The listing builds one solid part. Answer for the finished solid, in the listing's coordinates (mm). Give positions to 0.01 mm unless a question says otherwise; leave off trailing zeros. Loops run counter-clockwise (first coordinate to the right, second up) from the corner with the lowest first, then second, coordinate; pieces in that order, holes last. Notation, with made-up numbers: (67, 53.25) - (125, 53.25) arc R30 ccw to (125, 92.25) - close; hole circle Ø2 at (46.5, 77). An arc over 180 degrees is marked (long way). Answer in a Markdown table with one row per item. Add a question column.
```python
from build123d import *

# Parameters (mm, degrees)
SKETCH1_W           = 200
SKETCH1_H           = 180
BOSS_EXTRUDE1_DEPTH = 2
SKETCH2_W           = 55
SKETCH2_H           = 50
CUT_EXTRUDE1_DEPTH  = 4
SKETCH3_W           = 30
SKETCH3_H           = 70
CUT_EXTRUDE2_DEPTH  = 16
SKETCH4_R           = 1.5
CUT_EXTRUDE3_DEPTH  = 10
SKETCH5_R           = 1.75
CUT_EXTRUDE4_DEPTH  = 10
SKETCH6_R           = 1.5
CUT_EXTRUDE5_DEPTH  = 2
SKETCH7_R           = 1.15
CUT_EXTRUDE6_DEPTH  = 2
SKETCH8_R           = 1.5
CUT_EXTRUDE7_DEPTH  = 2


with BuildPart() as part:
    # Sketch1 → Boss-Extrude1 (new body)
    with BuildSketch(Plane(origin=(0, 0, 0), x_dir=(1, 0, 0), z_dir=(0, 1, 0))):
        Rectangle(SKETCH1_W, SKETCH1_H)
    extrude(amount=BOSS_EXTRUDE1_DEPTH)

    # Sketch2 → Cut-Extrude1 (cut)
    with BuildSketch(Plane(origin=(0, 2, 0), x_dir=(1, 0, 0), z_dir=(0, 1, 0))):
        with Locations((0.5, -65)):
            Rectangle(SKETCH2_W, SKETCH2_H)
    extrude(amount=-CUT_EXTRUDE1_DEPTH, mode=Mode.SUBTRACT)

    # Sketch3 → Cut-Extrude2 (cut)
    with BuildSketch(Plane(origin=(0, 2, 0), x_dir=(1, 0, 0), z_dir=(0, 1, 0))):
        with Locations((85, 55)):
            Rectangle(SKETCH3_W, SKETCH3_H)
        with Locations((-85, 55)):
            Rectangle(SKETCH3_W, SKETCH3_H)
    extrude(amount=-CUT_EXTRUDE2_DEPTH, mode=Mode.SUBTRACT)

    # Sketch4 → Cut-Extrude3 (cut)
    with BuildSketch(Plane(origin=(0, 2, 0), x_dir=(1, 0, 0), z_dir=(0, 1, 0))):
        with Locations((90, -80)):
            Circle(SKETCH4_R)
        with Locations((-90, -80)):
            Circle(SKETCH4_R)
        with Locations((60, 80)):
            Circle(SKETCH4_R)
        with Locations((-60, 80)):
            Circle(SKETCH4_R)
    extrude(amount=-CUT_EXTRUDE3_DEPTH, mode=Mode.SUBTRACT)

    # Sketch5 → Cut-Extrude4 (cut)
    with BuildSketch(Plane(origin=(0, 2, 0), x_dir=(1, 0, 0), z_dir=(0, 1, 0))):
        with Locations((60, 20)):
            Circle(SKETCH5_R)
        with Locations((22.6, 20)):
            Circle(SKETCH5_R)
        with Locations((22.6, -16.7)):
            Circle(SKETCH5_R)
        with Locations((60, -16.7)):
            Circle(SKETCH5_R)
    extrude(amount=-CUT_EXTRUDE4_DEPTH, mode=Mode.SUBTRACT)

    # Sketch6 → Cut-Extrude5 (cut)
    with BuildSketch(Plane(origin=(0, 2, 0), x_dir=(1, 0, 0), z_dir=(0, 1, 0))):
        with Locations((-95, -60.635083269)):
            Circle(SKETCH6_R)
        with Locations((-95, -18.235083269)):
            Circle(SKETCH6_R)
        with Locations((95, -60.635083269)):
            Circle(SKETCH6_R)
        with Locations((95, -18.235083269)):
            Circle(SKETCH6_R)
    extrude(amount=-CUT_EXTRUDE5_DEPTH, mode=Mode.SUBTRACT)

    # Sketch7 → Cut-Extrude6 (cut)
    with BuildSketch(Plane.XZ):
        with Locations((64, 40)):
            Circle(SKETCH7_R)
        with Locations((71.597678191, 28.840910158)):
            Circle(SKETCH7_R)
        with Locations((-64, 40)):
            Circle(SKETCH7_R)
        with Locations((-71.597678191, 28.840910158)):
            Circle(SKETCH7_R)
    extrude(amount=-CUT_EXTRUDE6_DEPTH, mode=Mode.SUBTRACT)

    # Sketch8 → Cut-Extrude7 (cut)
    with BuildSketch(Plane.XZ):
        with Locations((60.59, -62.42)):
            Circle(SKETCH8_R)
        with Locations((54.39, -62.42)):
            Circle(SKETCH8_R)
        with Locations((48.19, -62.42)):
            Circle(SKETCH8_R)
        with Locations((41.99, -62.42)):
            Circle(SKETCH8_R)
        with Locations((35.79, -62.42)):
            Circle(SKETCH8_R)
        with Locations((29.59, -62.42)):
            Circle(SKETCH8_R)
        with Locations((23.39, -62.42)):
            Circle(SKETCH8_R)
        with Locations((-23.39, -62.42)):
            Circle(SKETCH8_R)
        with Locations((-29.59, -62.42)):
            Circle(SKETCH8_R)
        with Locations((-35.79, -62.42)):
            Circle(SKETCH8_R)
        with Locations((-41.99, -62.42)):
            Circle(SKETCH8_R)
        with Locations((-60.59, -62.42)):
            Circle(SKETCH8_R)
        with Locations((-54.39, -62.42)):
            Circle(SKETCH8_R)
        with Locations((-48.19, -62.42)):
            Circle(SKETCH8_R)
    extrude(amount=-CUT_EXTRUDE7_DEPTH, mode=Mode.SUBTRACT)


solid = part.part
```
(1) A cutting plane is placed at A-A on x = -1. Determine the outline of the cut face in (y, z).
(2) A cutting plane is placed at C-C on y = 0.6. Give the number of separate pieces and of enclosed holes in the cut face, plus the area to 3 significant figures.
(3) Find the intervals of material crossed by line 1 along X through (y, z) = (0.5, 16.7); line 2 along X through (y, z) = (0.35, 82); line 3 along Z through (x, y) = (-54.39, 0.5), in increasing order. Write a range as [from, to].
(4) A cutting plane is placed at B-B on z = -24.5. Determine the outline of the cut face in (x, y).
(5) Given pin 1 Ø4 at (x, z) = (60, -80) entering from +Y; pin 2 Ø1 at (y, z) = (1.5, -31.5) entering from -X, each flat-ended and moving along its own axis, determine where each tip first touches the part or whether it passes through.
Evaluation:
| question | item | result |
|---|---|---|
| 1 | outline | (0, -90) - (2, -90) - (2, 40) - (0, 40) - close |
| 2 | separate pieces | 1 |
| 2 | enclosed holes | 30 |
| 2 | area | 28,800 mm² |
| 3 | line 1 | x = [-100, 20.85], [24.35, 58.25], [61.75, 100] |
| 3 | line 2 | x = [-100, -27], [28, 100] |
| 3 | line 3 | z = [-90, -63.92], [-60.92, 90] |
| 4 | outline | (-70, 0) - (70, 0) - (70, 2) - (-70, 2) - close |
| 5 | pin 1 | stops at y = 2 |
| 5 | pin 2 | stops at x = -70 |
